Could you check a few things on this drawing? It's one solid part, dimensions in mm from its lowest x, y, z. Give positions to 0.01 mm unless a question says otherwise; leave off trailing zeros. Order: outer loops, then holes, each group sorted by start corner. A loop starts at its lowest first (then second) coordinate and runs counter-clockwise, first axis right, second up. Notation, with made-up numbers: (46.25, -3.75) - (94.25, -3.75) arc R31 cw to (94.25, 35.25) - close; hole circle Ø2 at (-37, 47.5). An arc over 180 degrees is marked (long way). Return JSON: item names as keys, results as strings.
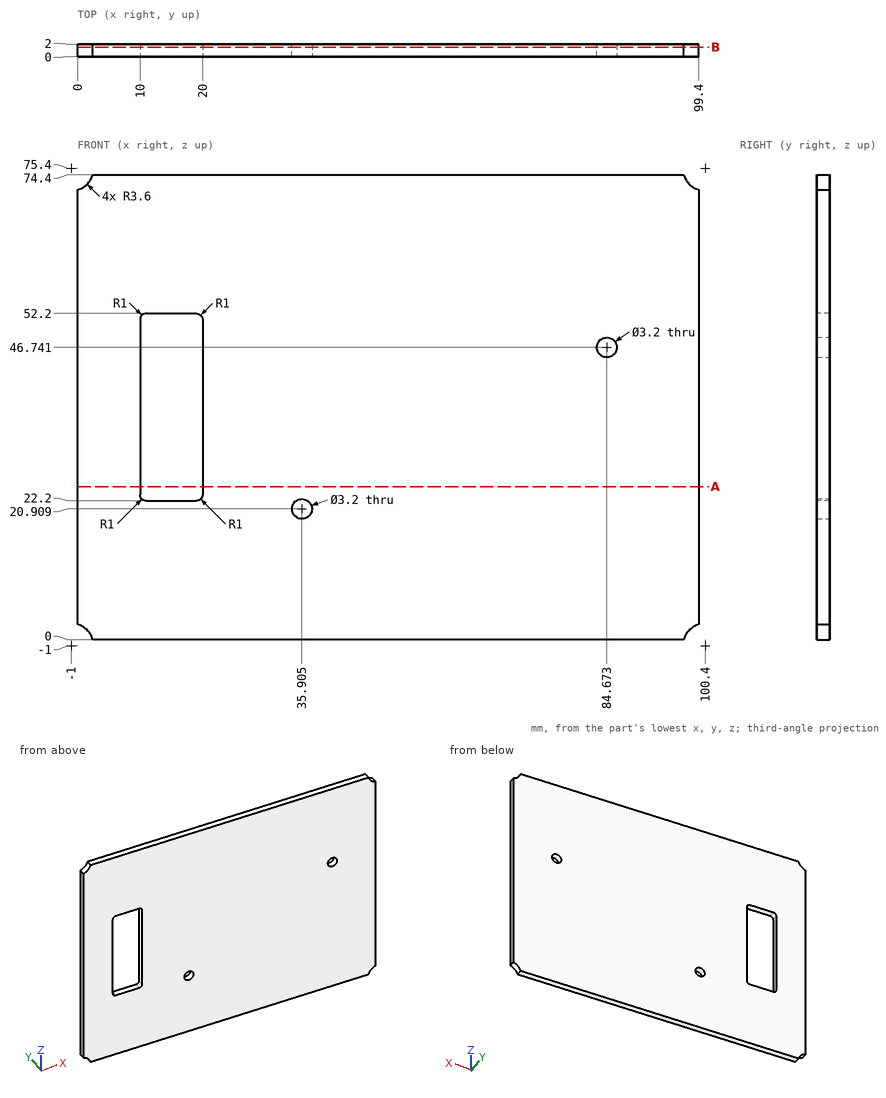
1. If I drill on L1, parallel to X at y = 0.5, z = 42.5; L2, parallel to X at y = 1.3, z = 46.5 (1 decimal); L3, parallel to Z at x = 13.5, y = 1.65, over which ranges is the centre line in solid material (lowest first)? Write a range as [from, to].
Checks:
{"L1": "[0, 10], [20, 99.4]", "L2": "[0, 10], [20, 83.1], [86.3, 99.4]", "L3": "[0, 22.2], [52.2, 74.4]"}
2. Suppose I cut it at A-A (z = 24.5). List the corners of the cut face in (x, y) for me, plus the area to 3 significant figures.
Checks:
{"outline": "(0, 0) - (10, 0) - (10, 2) - (0, 2) - close; (20, 0) - (99.4, 0) - (99.4, 2) - (20, 2) - close", "area": "179 mm^2"}
3. Suppose I cut it at B-B (y = 1.5). List the corners of the cut face in (x, z) for me (1 decimal).
Checks:
{"outline": "(0, 2.5) arc R3.6 cw to (2.5, 0) - (96.9, 0) arc R3.6 cw to (99.4, 2.5) - (99.4, 71.9) arc R3.6 cw to (96.9, 74.4) - (2.5, 74.4) arc R3.6 cw to (0, 71.9) - close; hole (10, 23.2) arc R1 ccw to (11, 22.2) - (19, 22.2) arc R1 ccw to (20, 23.2) - (20, 51.2) arc R1 ccw to (19, 52.2) - (11, 52.2) arc R1 ccw to (10, 51.2) - close; hole circle Ø3.2 at (35.9, 20.9); hole circle Ø3.2 at (84.7, 46.7)"}
